from build123d import *

# Parameters (mm, degrees)
BASE_FLANGE1_DEPTH   = 1.5875
EDGE_FLANGE1_START   = -23.8125
EDGE_FLANGE1_DEPTH   = 47.625
EDGE_FLANGE1_2_DEPTH = 47.625
SKETCH9_R            = 3.175
CUT_EXTRUDE1_DEPTH   = 2.54
CUT_EXTRUDE2_DEPTH   = 2.54


# Read off the part's stored shape, not the designer's step: Edge-Flange1
# Sheet-metal steps are written as plain solids
with BuildPart() as part:
    # Sketch1 → Base-Flange1 (new body)
    with BuildSketch(Plane(origin=(0, 285.976549587, -785.714112483), x_dir=(1, 0, 0), z_dir=(0, -0.34202014332566955, 0.9396926207859082))):
        with BuildLine():
            Line((-27.5, 159.361299231), (27.5, 159.361299231))
            ThreePointArc((27.5, 159.361299231), (36.907682688, 151.326645312), (30.443979637, 140.777678536))
            ThreePointArc((30.443979637, 140.777678536), (25.645376408, 137.290929389), (23.8125, 131.64960183))
            Line((23.8125, 131.64960183), (23.8125, 98.987567929))
            Line((23.8125, 98.987567929), (-23.8125, 98.987567929))
            Line((-23.8125, 98.987567929), (-23.8125, 131.64960183))
            ThreePointArc((-23.8125, 131.64960183), (-25.645376408, 137.290929389), (-30.443979637, 140.777678536))
            ThreePointArc((-30.443979637, 140.777678536), (-36.907682688, 151.326645312), (-27.5, 159.361299231))
        make_face()
    extrude(amount=BASE_FLANGE1_DEPTH)

    # Edge-Flange1 outline → Edge-Flange1 (cut)
    with BuildSketch(Plane.YZ.offset(EDGE_FLANGE1_START)):
        with BuildLine():
            Line((378.994436719, -751.858370313), (378.994436719, -751.849696253))
            ThreePointArc((378.994436719, -751.849696253), (379.428526068, -750.472940733), (380.573785769, -749.594152055))
            Line((380.573785769, -749.594152055), (378.451479742, -750.366608277))
            Line((378.451479742, -750.366608277), (378.994436719, -751.858370313))
        make_face()
    extrude(amount=EDGE_FLANGE1_DEPTH, mode=Mode.SUBTRACT)

    # Edge-Flange1 2 outline → Edge-Flange1 2 (add)
    with BuildSketch(Plane.YZ.offset(EDGE_FLANGE1_START)):
        with BuildLine():
            Line((381.116742747, -751.085914091), (378.994436719, -751.858370313))
            Line((378.994436719, -751.858370313), (378.994436719, -769.218988099))
            Line((378.994436719, -769.218988099), (380.581936719, -769.218988099))
            Line((380.581936719, -769.218988099), (380.581936719, -751.849696253))
            ThreePointArc((380.581936719, -751.849696253), (380.728929938, -751.383493326), (381.116742747, -751.085914091))
        make_face()
    extrude(amount=EDGE_FLANGE1_2_DEPTH)

    # Sketch9 → Cut-Extrude1 (cut)
    with BuildSketch(Plane(origin=(0, 285.433592609, -784.222350448), x_dir=(1, 0, 0), z_dir=(0, -0.34202014332566955, 0.9396926207859082))):
        with Locations(Location((-27.5, 149.836299231, 0), (0, 0, 270))):
            Circle(SKETCH9_R)
        with Locations(Location((27.5, 149.836299231, 0), (0, 0, 270))):
            Circle(SKETCH9_R)
    extrude(amount=-CUT_EXTRUDE1_DEPTH, mode=Mode.SUBTRACT)

    # Sketch10 → Cut-Extrude2 (cut)
    with BuildSketch(Plane(origin=(0, 285.976549587, -785.714112483), x_dir=(-1, 0, 0), z_dir=(0, 0.34202014332566955, -0.9396926207859082))):
        with BuildLine():
            Line((-11.1125, 153.011299231), (11.1125, 153.011299231))
            ThreePointArc((11.1125, 153.011299231), (15.602628061, 151.151427292), (17.4625, 146.661299231))
            Line((17.4625, 146.661299231), (17.4625, 110.77107883))
            ThreePointArc((17.4625, 110.77107883), (15.602628061, 106.28095077), (11.1125, 104.42107883))
            Line((11.1125, 104.42107883), (-11.1125, 104.42107883))
            ThreePointArc((-11.1125, 104.42107883), (-15.602628061, 106.28095077), (-17.4625, 110.77107883))
            Line((-17.4625, 110.77107883), (-17.4625, 146.661299231))
            ThreePointArc((-17.4625, 146.661299231), (-15.602628061, 151.151427292), (-11.1125, 153.011299231))
        make_face()
    extrude(amount=-CUT_EXTRUDE2_DEPTH, mode=Mode.SUBTRACT)


solid = part.part
Check sheet for the modelled part. Datum: model origin and axes. Units: mm. A direction names the side the tool comes from. Give positions to 0.01 mm unless a question says otherwise; leave off trailing zeros. Loops run counter-clockwise (first coordinate to the right, second up) from the corner with the lowest first, then second, coordinate; pieces in that order, holes last. Notation, with made-up numbers: M 18.25,64.25 L 22.25,64.25 A24 ccw 22.25,94.25 Z; hole C 72.25,-33.5 d4. An arc over 180 degrees is marked long. Use a Markdown table: item, result. Add a question column.
Q1. Tool access check on faces 1 (the flat face through (0, 380.582, -761)), 2 (the cylindrical face through (-15.553, 427.791, -733.265)), 3 (the cylindrical face through (-0.333, 379.417, -750.49)), 4 (the flat face through (0, 378.994, -760)), 5 (the cylindrical face through (-15.652, 385.627, -748.611)). Record the directions out of +Z, -Z, +X, -X, +Y, -Y that give a thin tool (end or side, any length) a straight path to the whole face; none if there is none.
Q2. Sectioned sample at B-B, the plane z = -742. Record the cut outline in (x, y).
Q3. Sectioned sample at D-D, the plane x = 22.5. Record the cut outline in (y, z).
Q4. Sectioned sample at A-A, the plane x = -8. Record the cut outline in (y, z).
Q5. Mould release check, pull along Y, two halves, no side actions. Record for faces 6 (the cylindrical face through (15.65, 427.7, -733.3)), 7 (the cylindrical face through (25.57, 428.87, -732.85)), 8 (the flat face through (2.915, 430.798, -733.003)): pulls with the +Y half, pulls with the -Y half, needs draft (parallel to the pull), parting line crosses it, or undercut.
Q6. Scan lines: line 1 along X through (y, z) = (388, -748); line 2 along Y through (x, z) = (9, -759); line 3 along Z through (x, y) = (-17.5, 403). Record each from-to range of solid material in increasing order. Write a range as [from, to].
Q7. Sectioned sample at C-C, the plane y = 406. Record the cut outline in (x, z).
Q8. Go/stop test with flat-tipped pins: pin 1 (8.5 mm diameter, centred on x = 7.5, z = -762.5, fed in from +Y); pin 2 (4 mm diameter, centred on x = -24, y = 408.5, fed in from -Z); pin 3 (15 mm diameter, centred on y = 396, z = -760.5, fed in from -X); pin 4 (5 mm diameter, centred on x = -18, y = 429, fed in from -Z). Record where each tip stops, or that it passes through.
Verdict:
| question | item | result |
|---|---|---|
| 1 | face 1 | -Z, +X, -X, +Y |
| 1 | face 2 | -Z, -Y |
| 1 | face 3 | +Z, +X, -X, -Y |
| 1 | face 4 | +Z, -Z, +X, -X, -Y |
| 1 | face 5 | +Z, +Y |
| 2 | outline | M -23.81,401.44 L -17.46,401.44 L -17.46,406.08 L -23.81,406.08 Z; M 17.46,401.44 L 23.81,401.44 L 23.81,406.08 L 17.46,406.08 Z |
| 3 | outline | M 378.99,-769.22 L 380.58,-769.22 L 380.58,-751.85 A0.81 cw 381.12,-751.09 L 435.73,-731.21 L 435.18,-729.72 L 380.57,-749.59 A2.4 ccw 378.99,-751.85 Z |
| 4 | outline | M 378.99,-769.22 L 380.58,-769.22 L 380.58,-751.85 A0.81 cw 381.12,-751.09 L 384.1,-750 L 383.56,-748.51 L 380.57,-749.59 A2.4 ccw 378.99,-751.85 Z; M 429.22,-731.89 L 429.76,-733.38 L 435.73,-731.21 L 435.18,-729.72 Z |
| 5 | face 6 | pulls with the -Y half |
| 5 | face 7 | undercut |
| 5 | face 8 | pulls with the +Y half |
| 6 | line 1 | [-23.81, -17.14], [17.14, 23.81] |
| 6 | line 2 | [378.99, 380.58] |
| 6 | line 3 | [-743.12, -741.43] |
| 7 | outline | M -23.81,-742.03 L -17.46,-742.03 L -17.46,-740.34 L -23.81,-740.34 Z; M 17.46,-742.03 L 23.81,-742.03 L 23.81,-740.34 L 17.46,-740.34 Z |
| 8 | pin 1 | y = 380.58 |
| 8 | pin 2 | z = -741.84 |
| 8 | pin 3 | through |
| 8 | pin 4 | z = -734.57 |
